from build123d import *

# Parameters (mm, degrees)
F0_R     = 4
F0_R_2   = 6.5
F0_R_3   = 49.5
F1_DEPTH = 10


# Not quite as in the source:
# - ends of sketch curves that miss each other by under 0.0002 mm in the source are joined


with BuildPart() as f1:
    # F0 (on Top) → F1 (new body)
    with BuildSketch(Plane.XY):
        with BuildLine():
            ThreePointArc((95.6705294551, -23.4392788665), (97.790074014, -11.804720426), (98.5, 0))
            ThreePointArc((98.5, 0), (97.790074014, 11.804720426), (95.6705294551, 23.4392788665))
            ThreePointArc((95.6705294551, 23.4392788665), (77.143947059, 31.9540684018), (84.2233479596, 51.0752010798))
            ThreePointArc((84.2233479596, 51.0752010798), (69.6500179469, 69.6500179469), (51.0752071036, 84.2233531708))
            ThreePointArc((51.0752071036, 84.2233531708), (31.9540684018, 77.143947059), (23.4392785061, 95.6705221617))
            ThreePointArc((23.4392785061, 95.6705221617), (0, 98.5), (-23.4392788665, 95.6705294551))
            ThreePointArc((-23.4392788665, 95.6705294551), (-22.8817314531, 93.3658702171), (-22.69432, 91.00214))
            ThreePointArc((-22.69432, 91.00214), (-34.2095830083, 76.4125338333), (-51.0752010798, 84.2233479596))
            ThreePointArc((-51.0752010798, 84.2233479596), (-69.6500179469, 69.6500179469), (-84.2233531708, 51.0752071036))
            ThreePointArc((-84.2233531708, 51.0752071036), (-78.2216528988, 45.5466540133), (-76.00214, 37.69432))
            ThreePointArc((-76.00214, 37.69432), (-82.1994623513, 25.5488325165), (-95.6705221617, 23.4392785061))
            ThreePointArc((-95.6705221617, 23.4392785061), (-98.5, 0), (-95.6705294551, -23.4392788665))
            ThreePointArc((-95.6705294551, -23.4392788665), (-82.1994623513, -25.5488325165), (-76.00214, -37.69432))
            ThreePointArc((-76.00214, -37.69432), (-78.2216493872, -45.5466482978), (-84.2233479596, -51.0752010798))
            ThreePointArc((-84.2233479596, -51.0752010798), (-69.6500179469, -69.6500179469), (-51.0752071036, -84.2233531708))
            ThreePointArc((-51.0752071036, -84.2233531708), (-34.2095830083, -76.4125338333), (-22.69432, -91.00214))
            ThreePointArc((-22.69432, -91.00214), (-22.8817303816, -93.3658635024), (-23.4392785061, -95.6705221617))
            ThreePointArc((-23.4392785061, -95.6705221617), (0, -98.5), (23.4392788665, -95.6705294551))
            ThreePointArc((23.4392788665, -95.6705294551), (31.9540745992, -77.143944492), (51.0752071429, -84.2233599276))
            ThreePointArc((51.0752071429, -84.2233599276), (69.6500179469, -69.6500179469), (84.2233531708, -51.0752071036))
            ThreePointArc((84.2233531708, -51.0752071036), (77.1439496611, -31.9540621197), (95.6705294551, -23.4392788665))
        make_face()
        with Locations((-62.9325, -62.9325)):
            Circle(F0_R, mode=Mode.SUBTRACT)
        with Locations((0, -89)):
            Circle(F0_R, mode=Mode.SUBTRACT)
        with Locations((0, -60.5)):
            Circle(F0_R_2, mode=Mode.SUBTRACT)
        with Locations((-89, 0)):
            Circle(F0_R, mode=Mode.SUBTRACT)
        with Locations((-60.5, 0)):
            Circle(F0_R_2, mode=Mode.SUBTRACT)
        Circle(F0_R_3, mode=Mode.SUBTRACT)
        with Locations((62.9325, -62.9325)):
            Circle(F0_R, mode=Mode.SUBTRACT)
        with Locations((60.5, 0)):
            Circle(F0_R_2, mode=Mode.SUBTRACT)
        with Locations((89, 0)):
            Circle(F0_R, mode=Mode.SUBTRACT)
        with Locations((-62.9325, 62.9325)):
            Circle(F0_R, mode=Mode.SUBTRACT)
        with Locations((0, 60.5)):
            Circle(F0_R_2, mode=Mode.SUBTRACT)
        with Locations((0, 89)):
            Circle(F0_R, mode=Mode.SUBTRACT)
        with Locations((62.9325, 62.9325)):
            Circle(F0_R, mode=Mode.SUBTRACT)
    extrude(amount=F1_DEPTH)


solid = f1.part
The model under review builds one solid part; all positions refer to its coordinate system, in mm. A direction names the side the tool comes from. Round coordinates to 2 decimals unless told otherwise and drop trailing zeros. Write each loop counter-clockwise with the first axis right and the second up, starting at its lowest first coordinate (ties: lowest second). Pieces come first, ordered by that corner, then holes. Notation, with made-up numbers: M -38.5,-39.75 L -12.5,-39.75 A25 cw -12.5,-5.75 Z; hole C -2,72.5 d5. An arc over 180 degrees is marked long. Answer as CSV lines item,"result". Start each with the question number.
Q1. Clearance check with flat-ended pins moving along their axes: P1, Ø1, axis at x = -56, z = 8, coming from the -Y side; P2, Ø1.5, axis at y = 75, z = 2, coming from the +X side; P3, Ø6.5, axis at x = 62.93, y = 62.93, coming from the -Z side; P4, Ø6, axis at x = -50, z = 3.5, coming from the -Y side. State where each tip first meets the part, or that it passes through.
Q2. Consider section D-D, the plane x = -89. Give the boundary of the cut face in (y, z).
Q3. Consider section B-B, the plane y = 81.5. Give the boundary of the cut face in (x, z), then the cut area to 3 significant figures.
Q4. Consider section A-A, the plane x = 0. Give the boundary of the cut face in (y, z), then the cut area to 3 significant figures.
Q5. The part is to be moulded in two halves that separate along Y. For faces 3 (the face through (-69.9, -69.4, 4.9)), 4 (the face through (-45, 23, 10)), 5 (the face through (62.07, -66.84, 4.93)), 6 (the face through (-98.5, 0.3, 4.9)), say which applies: +Y half, -Y half, draft (parallel to the pull), parting line (faces both ways), or undercut.
Q6. Tool access review of faces 1 (the face through (-78.28, 45.64, 4.93)), 2 (the face through (77.267, 31.665, 4.93)): name each direction out of +Z, -Z, +X, -X, +Y, -Y from which nothing blocks a thin tool from reaching the whole face with its end or side.
Q7. Wall thickness on line 1 along Y through (x, z) = (60.5, 2.75); line 2 along X through (y, z) = (5.5, 5.25); line 3 along Y through (x, z) = (6, 6): over which ranges is each line inside the solid? List them lowest first.
Result set:
1,P1,"stops at y = -81.38"
1,P2,"stops at x = 64.72"
1,P3,"passes through"
1,P4,"stops at y = -84.22"
2,outline,"M -22.83,0 L -4,0 L -4,10 L -22.83,10 Z; M 4,0 L 22.83,0 L 22.83,10 L 4,10 Z"
3,outline,"M -55.32,0 L -49.3,0 L -49.3,10 L -55.32,10 Z; M -26.09,0 L 26.09,0 L 26.09,10 L -26.09,10 Z; M 49.3,0 L 55.32,0 L 55.32,10 L 49.3,10 Z"
3,area,"642 mm²"
4,outline,"M -98.5,0 L -93,0 L -93,10 L -98.5,10 Z; M -85,0 L -67,0 L -67,10 L -85,10 Z; M -54,0 L -49.5,0 L -49.5,10 L -54,10 Z; M 49.5,0 L 54,0 L 54,10 L 49.5,10 Z; M 67,0 L 85,0 L 85,10 L 67,10 Z; M 93,0 L 98.5,0 L 98.5,10 L 93,10 Z"
4,area,"560 mm²"
5,face 3,"-Y half"
5,face 4,"draft"
5,face 5,"undercut"
5,face 6,"parting line"
6,face 1,"+Z, -Z, -X"
6,face 2,"+Z, -Z"
7,line 1,"y = -77.73 to -66.11, -59.76 to -6.5, 6.5 to 59.76, 66.11 to 77.73"
7,line 2,"x = -98.35 to -63.96, -57.04 to -49.19, 49.19 to 57.04, 63.96 to 98.35"
7,line 3,"y = -98.32 to -63, -58 to -49.14, 49.14 to 58, 63 to 98.32"
